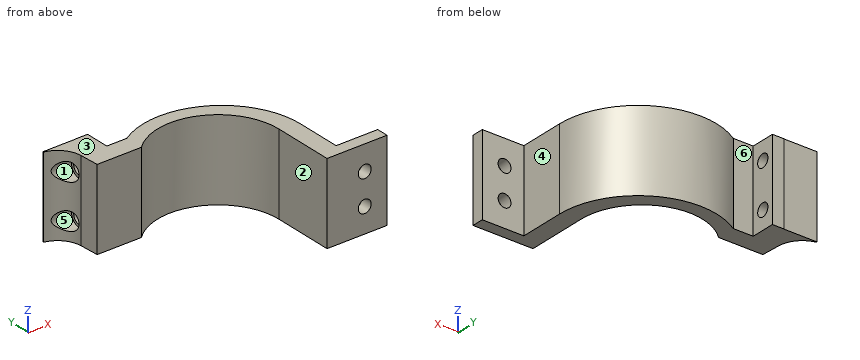
from build123d import *

# Parameters (mm, degrees)
BOSS_EXTRUDE1_DEPTH = 44
CUT_EXTRUDE1_REACH  = 8.35
SKETCH2_R           = 3.5
BOSS_EXTRUDE2_DEPTH = 44
CUT_EXTRUDE2_REACH  = 26.336
SKETCH5_R           = 3.5
SKETCH6_R           = 5
CUT_EXTRUDE3_DEPTH  = 15


with BuildPart() as part:
    # Sketch1 → Boss-Extrude1 (new body)
    with BuildSketch(Plane.XY):
        with BuildLine():
            Line((33.003348812, 0), (33.003348812, -33))
            Line((33.003348812, -33), (65.632108119, -33))
            Line((65.632108119, -33), (65.632108119, -26.65))
            Line((65.632108119, -26.65), (43.003348812, -26.65))
            Line((43.003348812, -26.65), (43.003348812, -2.369569967))
            ThreePointArc((43.003348812, -2.369569967), (20.809611253, 35.186501293), (-22.793831907, 33.859768466))
            Line((-22.793831907, 33.859768466), (-33.65, 33.859768466))
            Line((-33.65, 33.859768466), (-33.65, 46.995147616))
            Line((-33.65, 46.995147616), (-40, 46.995147616))
            Line((-40, 46.995147616), (-40, 23.859768466))
            Line((-40, 23.859768466), (-22.793831907, 23.859768466))
            ThreePointArc((-22.793831907, 23.859768466), (12.978190551, 30.342272193), (33.003348812, 0))
        make_face()
    extrude(amount=-BOSS_EXTRUDE1_DEPTH)

    # Sketch2 → Cut-Extrude1 (cut, up to next)
    with BuildSketch(Plane(origin=(0, -26.65, 0), x_dir=(1, 0, 0), z_dir=(0, 1, 0)), mode=Mode.PRIVATE) as cut_extrude1_sk1:
        with Locations((53.516422245, 13.5)):
            Circle(SKETCH2_R)
    cut_extrude1_tool1 = extrude(cut_extrude1_sk1.sketch, amount=-CUT_EXTRUDE1_REACH, mode=Mode.PRIVATE) & part.part
    add(cut_extrude1_tool1.solids().sort_by_distance((53.516422, -26.65, -13.5))[0], mode=Mode.SUBTRACT)
    # Sketch2 → Cut-Extrude1 (cut, up to next)
    with BuildSketch(Plane(origin=(0, -26.65, 0), x_dir=(1, 0, 0), z_dir=(0, 1, 0)), mode=Mode.PRIVATE) as cut_extrude1_sk2:
        with Locations((53.516422245, 30.5)):
            Circle(SKETCH2_R)
    cut_extrude1_tool2 = extrude(cut_extrude1_sk2.sketch, amount=-CUT_EXTRUDE1_REACH, mode=Mode.PRIVATE) & part.part
    add(cut_extrude1_tool2.solids().sort_by_distance((53.516422, -26.65, -30.5))[0], mode=Mode.SUBTRACT)

    # Sketch4 → Boss-Extrude2 (add)
    with BuildSketch(Plane.XY):
        with BuildLine():
            Line((-40, 23.859768466), (-46.838602468, 23.859768466))
            Line((-46.838602468, 23.859768466), (-47.380853546, 34.206535409))
            ThreePointArc((-47.380853546, 34.206535409), (-50.578394755, 42.184822071), (-57.98577318, 46.544646919))
            Line((-57.98577318, 46.544646919), (-57.98577318, 46.904796258))
            Line((-57.98577318, 46.904796258), (-47.376426292, 46.904796258))
            Line((-47.376426292, 46.904796258), (-40, 46.904796258))
            Line((-40, 46.904796258), (-40, 23.859768466))
        make_face()
    extrude(amount=-BOSS_EXTRUDE2_DEPTH)

    # Sketch5 → Cut-Extrude2 (cut, up to next)
    with BuildSketch(Plane(origin=(-33.65, 0, 0), x_dir=(0, 0, -1), z_dir=(1, 0, 0)), mode=Mode.PRIVATE) as cut_extrude2_sk1:
        with Locations((10, 40.425147616)):
            Circle(SKETCH5_R)
    cut_extrude2_tool1 = extrude(cut_extrude2_sk1.sketch, amount=-CUT_EXTRUDE2_REACH, mode=Mode.PRIVATE) & part.part
    add(cut_extrude2_tool1.solids().sort_by_distance((-33.65, 40.425148, -10))[0], mode=Mode.SUBTRACT)
    # Sketch5 → Cut-Extrude2 (cut, up to next)
    with BuildSketch(Plane(origin=(-33.65, 0, 0), x_dir=(0, 0, -1), z_dir=(1, 0, 0)), mode=Mode.PRIVATE) as cut_extrude2_sk2:
        with Locations((34, 40.425147616)):
            Circle(SKETCH5_R)
    cut_extrude2_tool2 = extrude(cut_extrude2_sk2.sketch, amount=-CUT_EXTRUDE2_REACH, mode=Mode.PRIVATE) & part.part
    add(cut_extrude2_tool2.solids().sort_by_distance((-33.65, 40.425148, -34))[0], mode=Mode.SUBTRACT)

    # Sketch6 → Cut-Extrude3 (cut)
    with BuildSketch(Plane(origin=(-58.65, 0, 0), x_dir=(0, 0, -1), z_dir=(1, 0, 0))):
        with Locations((34, 40.425147616)):
            Circle(SKETCH6_R)
        with Locations((10, 40.425147616)):
            Circle(SKETCH6_R)
    extrude(amount=CUT_EXTRUDE3_DEPTH, mode=Mode.SUBTRACT)


solid = part.part
Work out the finished part from the listing and answer in its coordinate system (mm). Face numbers are marked on the shaded views. A direction names the side the tool comes from. Give positions to 0.01 mm unless a question says otherwise; leave off trailing zeros. Loops run counter-clockwise (first coordinate to the right, second up) from the corner with the lowest first, then second, coordinate; pieces in that order, holes last. Notation, with made-up numbers: (55.25, 79) - (109.25, 79) arc R22 ccw to (109.25, 106) - close; hole circle Ø7 at (62, 41.5). An arc over 180 degrees is marked (long way). Answer in a Markdown table with one row per item. Add a question column.
Q1. The part is cut by section B-B (x = -38). Determine the outline of the cut face in (y, z), and give its area (3 significant figures).
Q2. Determine the mould class of the marked faces 1, 2 and 3 for opening direction Z: released by +Z, released by -Z, zero draft, split by the parting line, or undercut.
Q3. The part is cut by section D-D (x = 4). Determine the outline of the cut face in (y, z), and give its area (3 significant figures).
Q4. The part is cut by section C-C (y = 3.5). Determine the outline of the cut face in (x, z), and give its area (3 significant figures).
Q5. A tool of negligible diameter and unlimited length cuts with its end or side. For the marked faces 4, 5 and 6, from which of +Z, -Z, +X, -X, +Y, -Y can it reach the whole face along a straight path? Write none if from no direction.
Q6. Each of these flat-tipped pins is pushed along its axis until it touches: P1, Ø8, axis at y = 20.5, z = -21, coming from the +X side; P2, Ø10, axis at x = -8, z = -27.5, coming from the -Y side; P3, Ø12, axis at y = -12, z = -21.5, coming from the +X side. Where does it stop, or does it pass through?
Q7. The part is cut by section A-A (z = -22). Determine the outline of the cut face in (x, y).
Q8. Consider line 1 along X through (y, z) = (-31.5, -30.5); line 2 along Y through (x, z) = (-40.25, -10); line 3 along Y through (x, z) = (-39, -34). Determine where each line is inside the solid, lowest interval first.
Solution:
| question | item | result |
|---|---|---|
| 1 | outline | (23.86, -44) - (47, -44) - (47, 0) - (23.86, 0) - close; hole circle Ø7 at (40.43, -34); hole circle Ø7 at (40.43, -10) |
| 1 | area | 941 mm² |
| 2 | face 1 | undercut |
| 2 | face 2 | zero draft |
| 2 | face 3 | released by +Z |
| 3 | outline | (32.76, -44) - (40.33, -44) - (40.33, 0) - (32.76, 0) - close |
| 3 | area | 333 mm² |
| 4 | outline | (32.82, -44) - (42.6, -44) - (42.6, 0) - (32.82, 0) - close |
| 4 | area | 430 mm² |
| 5 | face 4 | +Z, -Z, +X, +Y |
| 5 | face 5 | -X |
| 5 | face 6 | +Z, -Z, +Y |
| 6 | P1 | stops at x = 38.63 |
| 6 | P2 | stops at y = 30.33 |
| 6 | P3 | stops at x = 43 |
| 7 | outline | (-57.99, 46.54) arc R13.31 cw to (-47.38, 34.21) - (-46.84, 23.86) - (-22.79, 23.86) arc R33 cw to (33, 0) - (33, -33) - (65.63, -33) - (65.63, -26.65) - (43, -26.65) - (43, -2.37) arc R42.87 ccw to (-22.79, 33.86) - (-33.65, 33.86) - (-33.65, 47) - (-40, 47) - (-40, 46.9) - (-57.99, 46.9) - close |
| 8 | line 1 | x = 33 to 50.02, 57.02 to 65.63 |
| 8 | line 2 | y = 23.86 to 36.93, 43.93 to 46.9 |
| 8 | line 3 | y = 23.86 to 36.93, 43.93 to 47 |
